```python
from build123d import *

# Parameters (mm, degrees)
F0_W     = 304.8
F0_H     = 203.2
F1_DEPTH = 76.2
F2_R     = 1
F3_T     = -1.3
F4_R     = 5.5
F5_DEPTH = 76.201


with BuildPart() as f1:
    # F0 (on Top) → F1 (new body)
    with BuildSketch(Plane.XY):
        Rectangle(F0_W, F0_H)
    extrude(amount=F1_DEPTH)

    # F2
    f2_edges = [f1.edges().sort_by_distance(p)[0] for p in [
        (0, -101.6, 76.2),
        (-152.4, -101.6, 38.1),
        (-152.4, 0, 76.2),
        (152.4, 0, 76.2),
        (0, 101.6, 76.2),
        (152.4, 101.6, 38.1),
        (152.4, -101.6, 38.1),
        (-152.4, 101.6, 38.1),
    ]]
    fillet(f2_edges, radius=F2_R)

    # F3
    f3_openings = [f1.faces().sort_by_distance(p)[0] for p in [
        (0, 0, 0),
    ]]
    offset(amount=F3_T, openings=f3_openings)

    # F4 (on face) → F5 (cut, through all)
    with BuildSketch(Plane.XY.offset(76.2)):
        with Locations((-141.821339, 0)):
            Circle(F4_R)
        with Locations((-128.321339, 0)):
            Circle(F4_R)
        with Locations((-114.821339, 0)):
            Circle(F4_R)
        with Locations((-101.321339, 0)):
            Circle(F4_R)
        with Locations((-87.821339, 0)):
            Circle(F4_R)
        with Locations((-74.321339, 0)):
            Circle(F4_R)
        with Locations((-60.821339, 0)):
            Circle(F4_R)
        with Locations((-47.321339, 0)):
            Circle(F4_R)
        with Locations((-33.821339, 0)):
            Circle(F4_R)
        with Locations((-20.321339, 0)):
            Circle(F4_R)
        with Locations((-6.821339, 0)):
            Circle(F4_R)
        with Locations((6.678661, 0)):
            Circle(F4_R)
        with Locations((20.178661, 0)):
            Circle(F4_R)
        with Locations((33.678661, 0)):
            Circle(F4_R)
        with Locations((47.178661, 0)):
            Circle(F4_R)
        with Locations((60.678661, 0)):
            Circle(F4_R)
        with Locations((74.178661, 0)):
            Circle(F4_R)
        with Locations((87.678661, 0)):
            Circle(F4_R)
        with Locations((101.178661, 0)):
            Circle(F4_R)
        with Locations((114.678661, 0)):
            Circle(F4_R)
        with Locations((128.178661, 0)):
            Circle(F4_R)
        with Locations((141.678661, 0)):
            Circle(F4_R)
    extrude(amount=-F5_DEPTH, mode=Mode.SUBTRACT)


solid = f1.part
```
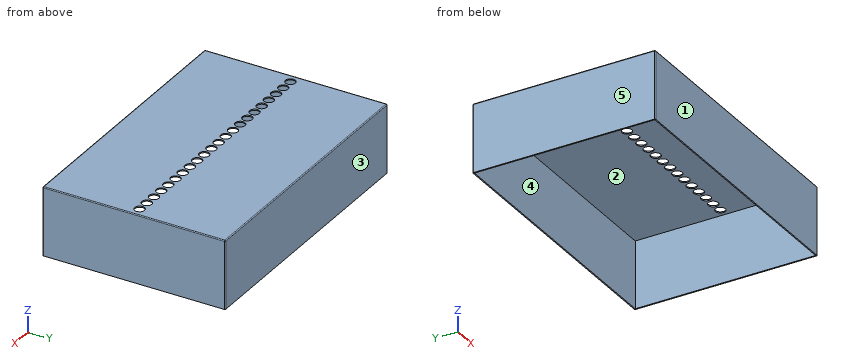
Geometry: final body of the model. Coordinates: model frame, mm. Face numbers are marked on the shaded views. A direction names the side the tool comes from. Coordinates: 2 decimals unless noted, no trailing zeros. Write each loop counter-clockwise with the first axis right and the second up, starting at its lowest first coordinate (ties: lowest second). Pieces come first, ordered by that corner, then holes. Notation, with made-up numbers: M 55.25,-29.75 L 74.25,-29.75 A13 cw 74.25,-10.75 Z; hole C 84.5,-2 d1. An arc over 180 degrees is marked long. Use CSV: the item, a comma, the result in double quotes. Start each with the question number.
1. Cut plane A-A on z = 34. Return the cut outline in (x, y), plus the area to 3 significant figures.
2. Ray query, probe 1 along X at (y, z) = (-23.5, 11.5); probe 2 along Y at (x, z) = (28, 23); probe 3 along Z at (x, y) = (77, 46.5). Return the intervals inside material, ascending.
3. Mould query, pull axis Y, two halves, no side actions, for the marked faces 3, 4 and 5. Classes: pulls with the +Y half, pulls with the -Y half, needs draft (parallel to the pull), parting line crosses it, or undercut.
4. First-contact query: P1, Ø12.5, axis at x = -60.82, y = 0, coming from the -Z side; P2, Ø6.5, axis at x = -20.32, y = 0, coming from the -Z side. Flat tips, straight axial feed; report the tip coordinate or a pass-through.
5. Cut plane D-D on y = 0. Count the separate pieces of the cut face and the enclosed holes in it, plus the area to 3 significant figures.
6. Cut plane B-B on y = 74. Return the cut outline in (x, z).
7. Reachability of the marked faces 1 and 2 from +Z, -Z, +X, -X, +Y, -Y: full face, straight path, thin tool, end or side. Return the list, or none.
8. Cut plane C-C on x = -34. Return the cut outline in (y, z).
Entries:
1,outline,"M -152.4,-100.6 A1 ccw -151.4,-101.6 L 151.4,-101.6 A1 ccw 152.4,-100.6 L 152.4,100.6 A1 ccw 151.4,101.6 L -151.4,101.6 A1 ccw -152.4,100.6 Z; hole M -151.1,-100.3 L 151.1,-100.3 L 151.1,100.3 L -151.1,100.3 Z"
1,area,"1,310 mm²"
2,probe 1,"-152.4 to -151.1, 151.1 to 152.4"
2,probe 2,"-101.6 to -100.3, 100.3 to 101.6"
2,probe 3,"74.9 to 76.2"
3,face 3,"pulls with the +Y half"
3,face 4,"undercut"
3,face 5,"needs draft"
4,P1,"z = 74.9"
4,P2,"through"
5,separate pieces,"23"
5,enclosed holes,"0"
5,area,"276 mm²"
6,outline,"M -152.4,0 L -151.1,0 L -151.1,74.9 L 151.1,74.9 L 151.1,0 L 152.4,0 L 152.4,75.2 A1 ccw 151.4,76.2 L -151.4,76.2 A1 ccw -152.4,75.2 Z"
7,face 1,"+Z, -Z, +X, -X, -Y"
7,face 2,"-Z"
8,outline,"M -101.6,0 L -100.3,0 L -100.3,74.9 L -5.5,74.9 L -5.5,76.2 L -100.6,76.2 A1 ccw -101.6,75.2 Z; M 5.5,74.9 L 100.3,74.9 L 100.3,0 L 101.6,0 L 101.6,75.2 A1 ccw 100.6,76.2 L 5.5,76.2 Z"
